```python
from build123d import *

# Parameters (mm, degrees)
EXTRUDE_1_DEPTH      = 100
SKETCH_4_R           = 1.6
CUT_EXTRUDE_7_DEPTH  = 124.99697577
SKETCH_7_R           = 19
CUT_EXTRUDE_8_DEPTH  = 61
SKETCH_3_R           = 1.6
CUT_EXTRUDE_9_DEPTH  = 124.99697577
SKETCH_5_R           = 19
CUT_EXTRUDE_10_DEPTH = 61


with BuildPart() as part:
    # 草图1 → 凸台-拉伸1 (new body)
    with BuildSketch(Plane(origin=(0, 0, 0), x_dir=(1, 0, 0), z_dir=(0, 1, 0))):
        with BuildLine():
            Line((-27.5, 31.5), (27.5, 31.5))
            ThreePointArc((27.5, 31.5), (34.571067812, 28.571067812), (37.5, 21.5))
            Line((37.5, 21.5), (37.5, -21.5))
            ThreePointArc((37.5, -21.5), (34.571067812, -28.571067812), (27.5, -31.5))
            Line((27.5, -31.5), (-27.5, -31.5))
            ThreePointArc((-27.5, -31.5), (-34.571067812, -28.571067812), (-37.5, -21.5))
            Line((-37.5, -21.5), (-37.5, 21.5))
            ThreePointArc((-37.5, 21.5), (-34.571067812, 28.571067812), (-27.5, 31.5))
        make_face()
    extrude(amount=-EXTRUDE_1_DEPTH)

    # 草图4 → 切除-拉伸7 (cut, through all)
    with BuildSketch(Plane(origin=(0, 0, -31.5), x_dir=(-1, 0, 0), z_dir=(0, 0, -1))):
        with Locations((0, -90.500000002)):
            Circle(SKETCH_4_R)
        with Locations((13.42339376, -82.750000001)):
            Circle(SKETCH_4_R)
        with BuildLine():
            ThreePointArc((7, -81.427584506), (11.429921133, -79.657213904), (13.419546961, -75.321340016))
            ThreePointArc((13.419546961, -75.321340016), (13.42339376, -75), (13.419546961, -74.678659984))
            ThreePointArc((13.419546961, -74.678659984), (11.429921133, -70.342786096), (7, -68.572415494))
            Line((7, -68.572415494), (-7, -68.572415494))
            ThreePointArc((-7, -68.572415494), (-11.429921133, -70.342786096), (-13.419546961, -74.678659984))
            ThreePointArc((-13.419546961, -74.678659984), (-13.42339376, -75), (-13.419546961, -75.321340016))
            ThreePointArc((-13.419546961, -75.321340016), (-11.429921133, -79.657213904), (-7, -81.427584506))
            Line((-7, -81.427584506), (7, -81.427584506))
        make_face()
        with Locations((-13.42339376, -82.750000001)):
            Circle(SKETCH_4_R)
        with Locations((13.42339376, -67.249999999)):
            Circle(SKETCH_4_R)
        with Locations((-13.42339376, -67.249999999)):
            Circle(SKETCH_4_R)
        with Locations((0, -59.499999998)):
            Circle(SKETCH_4_R)
    extrude(amount=-CUT_EXTRUDE_7_DEPTH, mode=Mode.SUBTRACT)

    # 草图7 → 切除-拉伸8 (cut)
    with BuildSketch(Plane(origin=(0, 0, -31.5), x_dir=(-1, 0, 0), z_dir=(0, 0, -1))):
        with Locations((0, -75)):
            Circle(SKETCH_7_R)
    extrude(amount=-CUT_EXTRUDE_8_DEPTH, mode=Mode.SUBTRACT)

    # 草图3 → 切除-拉伸9 (cut, through all)
    with BuildSketch(Plane.XY.offset(31.5)):
        with Locations((0.004610011, -41.094795393)):
            Circle(SKETCH_3_R)
        with Locations((13.428003771, -33.344795392)):
            Circle(SKETCH_3_R)
        with BuildLine():
            ThreePointArc((7.004610011, -32.022379898), (11.434531144, -30.252009295), (13.424156972, -25.916135407))
            ThreePointArc((13.424156972, -25.916135407), (13.428003771, -25.594795392), (13.424156972, -25.273455376))
            ThreePointArc((13.424156972, -25.273455376), (11.434531144, -20.937581488), (7.004610011, -19.167210885))
            Line((7.004610011, -19.167210885), (-6.995389989, -19.167210885))
            ThreePointArc((-6.995389989, -19.167210885), (-11.425311121, -20.937581488), (-13.414936949, -25.273455376))
            ThreePointArc((-13.414936949, -25.273455376), (-13.418783749, -25.594795392), (-13.414936949, -25.916135407))
            ThreePointArc((-13.414936949, -25.916135407), (-11.425311121, -30.252009295), (-6.995389989, -32.022379898))
            Line((-6.995389989, -32.022379898), (7.004610011, -32.022379898))
        make_face()
        with Locations((-13.418783749, -33.344795392)):
            Circle(SKETCH_3_R)
        with Locations((13.428003771, -17.844795391)):
            Circle(SKETCH_3_R)
        with Locations((-13.418783749, -17.844795391)):
            Circle(SKETCH_3_R)
        with Locations((0.004610011, -10.09479539)):
            Circle(SKETCH_3_R)
    extrude(amount=-CUT_EXTRUDE_9_DEPTH, mode=Mode.SUBTRACT)

    # 草图5 → 切除-拉伸10 (cut)
    with BuildSketch(Plane.XY.offset(31.5)):
        with Locations((0, -25)):
            Circle(SKETCH_5_R)
    extrude(amount=-CUT_EXTRUDE_10_DEPTH, mode=Mode.SUBTRACT)


solid = part.part
```
Part model, mm, in its own coordinate system. A direction names the side the tool comes from. Coordinates: 2 decimals unless noted, no trailing zeros. Write each loop counter-clockwise with the first axis right and the second up, starting at its lowest first coordinate (ties: lowest second). Pieces come first, ordered by that corner, then holes.
Item 1: Slice it at B-B (z = -4.5). Write the cut outline in (x, y).
Item 2: Which spindle directions (+Z, -Z, +X, -X, +Y, -Y) get a long thin tool onto all of the face, cutting with end or side? Do faces 1 (the face through (11.48, -79.61, 30.49)), 2 (the face through (0, -16, -29.5)), 3 (the face through (0, -83, 29.5)). Say none if no direction does.
Item 3: Slice it at A-A (y = -90.5). Write the cut outline in (x, z).
Item 4: Probe line 1 (Y direction, x = 0, z = 3); line 2 (Y direction, x = -1.5, z = -12.5); line 3 (Z direction, x = 9, y = -68.5). List the from-to ranges inside material, lowest first.
Item 5: Pin check, flat tips, straight feed: pin 1 (1.9 mm diameter, centred on x = -13.42, y = -17.84, fed in from +Z); pin 2 (5 mm diameter, centred on x = 0, y = -41.09, fed in from +Z); pin 3 (5 mm diameter, centred on x = 0, y = -90.5, fed in from -Z). Stop position of each tip, or through.
Item 6: Mould opens along X. For faces 4 (the face through (12.69, -84.17, 30.49)), 5 (the face through (0, -49, 31.5)), 6 (the face through (37.5, -49, 0)) say: released by +X, released by -X, zero draft, split by the parting line, or undercut.
Item 7: Slice it at C-C (x = 0). Count the separate pieces of the cut face and the enclosed holes in it, and give its area (3 significant figures).
Item 8: Slice it at D-D (y = -47). Write the cut outline in (x, z), and give its area (3 significant figures).
Results found:
1. outline: (-37.5, -100) - (37.5, -100) - (37.5, 0) - (-37.5, 0) - close; hole circle Ø38 at (0, -75); hole circle Ø38 at (0, -25)
2. face 1: +Z, -Z
2. face 2: +Z
2. face 3: -Z
3. outline: (-37.5, -21.5) arc R10 ccw to (-27.5, -31.5) - (-10.99, -31.5) - (-10.99, 29.5) - (-1.6, 29.5) - (-1.6, 31.5) - (-27.5, 31.5) arc R10 ccw to (-37.5, 21.5) - close; (1.6, 29.5) - (10.99, 29.5) - (10.99, -31.5) - (27.5, -31.5) arc R10 ccw to (37.5, -21.5) - (37.5, 21.5) arc R10 ccw to (27.5, 31.5) - (1.6, 31.5) - close
4. line 1: y = -100 to -94, -56 to -44, -6 to 0
4. line 2: y = -100 to -93.94, -56.06 to -43.94, -6.06 to 0
4. line 3: z = 29.5 to 31.5
5. pin 1: passes through
5. pin 2: stops at z = -29.5
5. pin 3: stops at z = 29.5
6. face 4: undercut
6. face 5: zero draft
6. face 6: released by +X
7. separate pieces: 7
7. enclosed holes: 0
7. area: 1,590 mm2
8. outline: (-37.5, -21.5) arc R10 ccw to (-27.5, -31.5) - (27.5, -31.5) arc R10 ccw to (37.5, -21.5) - (37.5, 21.5) arc R10 ccw to (27.5, 31.5) - (-27.5, 31.5) arc R10 ccw to (-37.5, 21.5) - close
8. area: 4,640 mm2
